from build123d import *

# Parameters (mm, degrees)
SKETCH4_W               = 22.352
SKETCH4_H               = 30.48
BOSS_EXTRUDE2_DEPTH     = 104.14
CUT_EXTRUDE2_START      = -100.33
SKETCH5_R               = 5.08
CUT_EXTRUDE2_DEPTH      = 100.33
CUT_EXTRUDE5_REACH      = 111.083
CUT_EXTRUDE5_END_RADIUS = 5.08
SKETCH9_R               = 4.445
LPATTERN1_COUNT         = 5
LPATTERN1_PITCH         = 16.51
SKETCH14_R              = 7.14375
CUT_EXTRUDE7_DEPTH      = 20.066


with BuildPart() as part:
    # Sketch4 → Boss-Extrude2 (new body)
    with BuildSketch(Plane(origin=(0, 0, 0), x_dir=(0, 0, -1), z_dir=(1, 0, 0))):
        Rectangle(SKETCH4_W, SKETCH4_H)
    extrude(amount=BOSS_EXTRUDE2_DEPTH)

    # Sketch5 → Cut-Extrude2 (cut)
    with BuildSketch(Plane.ZY.offset(CUT_EXTRUDE2_START)):
        with Locations((0, -1.9939)):
            Circle(SKETCH5_R)
    extrude(amount=CUT_EXTRUDE2_DEPTH, mode=Mode.SUBTRACT)

    # Cut-Extrude5: up to this cylinder (the profile starts outside it)
    cut_extrude5_end = Plane(origin=(28.321, -1.9939, 0), z_dir=(-1, 0, 0)) * Cylinder(CUT_EXTRUDE5_END_RADIUS, 233.326, mode=Mode.PRIVATE)
    # Sketch9 → Cut-Extrude5 (cut, up to the surface)
    with BuildSketch(Plane(origin=(0, 15.24, 0), x_dir=(1, 0, 0), z_dir=(0, 1, 0)), mode=Mode.PRIVATE) as cut_extrude5_sk1:
        with Locations(Location((28.321, 0, 0), (0, 0, 270))):
            Circle(SKETCH9_R)
    cut_extrude5_tool1 = extrude(cut_extrude5_sk1.sketch, amount=-CUT_EXTRUDE5_REACH, mode=Mode.PRIVATE) - cut_extrude5_end
    cut_extrude5 = cut_extrude5_tool1.solids().sort_by_distance((28.321, 15.24, 0))[0]
    add(cut_extrude5, mode=Mode.SUBTRACT)

    # LPattern1: Cut-Extrude5 ×5
    with Locations(*[(i * LPATTERN1_PITCH, 0, 0) for i in range(1, LPATTERN1_COUNT)]):
        add(cut_extrude5, mode=Mode.SUBTRACT)

    # Sketch14 → Cut-Extrude7 (cut)
    with BuildSketch(Plane.ZY):
        with Locations((0, -1.9939)):
            Circle(SKETCH14_R)
    extrude(amount=-CUT_EXTRUDE7_DEPTH, mode=Mode.SUBTRACT)


solid = part.part
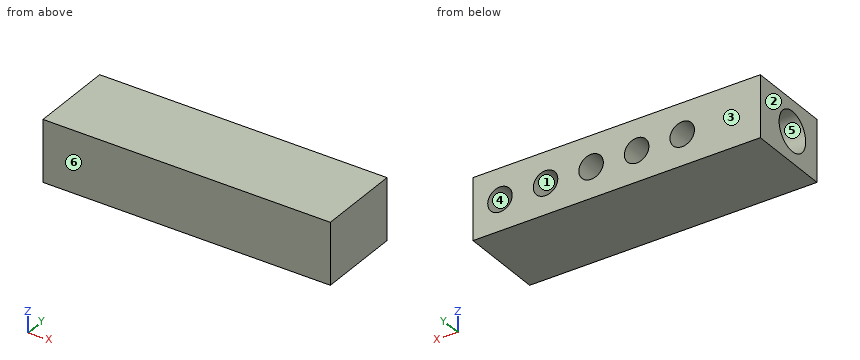
Geometry: final body of the model. Coordinates: model frame, mm. Face numbers are marked on the shaded views. A direction names the side the tool comes from. Round coordinates to 2 decimals unless told otherwise and drop trailing zeros. Loops run counter-clockwise (first coordinate to the right, second up) from the corner with the lowest first, then second, coordinate; pieces in that order, holes last. Notation, with made-up numbers: M 0,8.25 L 31,8.25 A26 cw 31,27.25 Z; hole C -3.75,20.25 d7. An arc over 180 degrees is marked long. One line per question, with ' | ' between items.
(1) Pull-direction query (X, two-part tool) for the marked faces 1, 2 and 3; classes: +X half, -X half, draft (parallel to the pull), parting line (faces both ways), or undercut.
Check result:
face 1: undercut | face 2: -X half | face 3: draft
(2) Access query for the marked faces 4, 5 and 6. Directions: +Z, -Z, +X, -X, +Y, -Y. A direction counts if a zero-diameter tool reaches every point of the face in a straight line with its end or side. Return the directions, or none.
Check result:
face 4: +Y | face 5: -X | face 6: +Z, -Z, +X, -X, -Y
(3) Cut plane B-B on y = 4. Return the cut outline in (x, z) (3 decimals).
Check result:
outline: M 0,-11.176 L 104.14,-11.176 L 104.14,11.176 L 0,11.176 L 0,3.887 L 20.066,3.887 L 20.066,-3.887 L 0,-3.887 Z; hole C 28.321,0 d8.89; hole C 44.831,0 d8.89; hole C 61.341,0 d8.89; hole C 77.851,0 d8.89; hole C 94.361,0 d8.89
(4) Material intervals for line 1 along X through (y, z) = (7.75, 0); line 2 along X through (y, z) = (3.75, 0); line 3 along Y through (x, z) = (6, 0), sorted ascending. Write a range as from..to.
Check result:
line 1: x = 0..23.88, 32.77..40.39, 49.28..56.9, 65.79..73.41, 82.3..89.92, 98.81..104.14 | line 2: x = 20.07..23.88, 32.77..40.39, 49.28..56.9, 65.79..73.41, 82.3..89.92, 98.81..104.14 | line 3: y = -15.24..-9.14, 5.15..15.24
(5) Cut plane C-C on x = 31.5. Return the cut outline in (y, z).
Check result:
outline: M -15.24,-11.18 L 15.24,-11.18 L 15.24,-3.11 L 2.03,-3.11 A5.08 cw long 2.03,3.11 L 15.24,3.11 L 15.24,11.18 L -15.24,11.18 Z
(6) Cut plane A-A on z = 0. Give the number of separate pieces and of enclosed holes in the cut face, plus the area to 3 significant figures.
Check result:
separate pieces: 6 | enclosed holes: 0 | area: 1,530 mm2
(7) Contact query for flat-ended pins moving along their axis: P1, Ø7, axis at x = 61.341, z = 0, coming from the +Y side; P2, Ø5.5, axis at x = 94.361, z = 0, coming from the +Y side. Output: stop coordinate, or through.
Check result:
P1: stops at y = -5.68 | P2: stops at y = -6.27
(8) Cut plane D-D on x = 6. Return the cut outline in (y, z), plus the area to 3 significant figures.
Check result:
outline: M -15.24,-11.18 L 15.24,-11.18 L 15.24,11.18 L -15.24,11.18 Z; hole C -1.99,0 d14.29 | area: 521 mm2
